from build123d import *

# Parameters (mm, degrees)
F0_R     = 3
F1_DEPTH = 10


with BuildPart() as f1:
    # F0 (on Top) → F1 (new body)
    with BuildSketch(Plane.XY):
        with BuildLine():
            ThreePointArc((4.242641, -1.5), (4.435194, -0.760959), (4.5, 0))
            ThreePointArc((4.5, 0), (4.435194, 0.760959), (4.242641, 1.5))
            ThreePointArc((4.242641, 1.5), (-4.5, 0), (4.242641, -1.5))
        make_face()
        Circle(F0_R, mode=Mode.SUBTRACT)
        with BuildLine():
            ThreePointArc((4.242641, 1.5), (4.435194, 0.760959), (4.5, 0))
            ThreePointArc((4.5, 0), (4.435194, -0.760959), (4.242641, -1.5))
            Line((4.242641, -1.5), (11.25223, -1.5))
            ThreePointArc((11.25223, -1.5), (11.161904, 0), (11.25223, 1.5))
            Line((11.25223, 1.5), (4.242641, 1.5))
        make_face()
    extrude(amount=F1_DEPTH)


solid = f1.part
Build history of the part. All positions in model axes, mm. A direction names the side the tool comes from. Give positions to 0.01 mm unless a question says otherwise; leave off trailing zeros. Write each loop counter-clockwise with the first axis right and the second up, starting at its lowest first coordinate (ties: lowest second). Pieces come first, ordered by that corner, then holes. Notation, with made-up numbers: (36.25, -2) - (60.25, -2) arc R22 cw to (60.25, 9) - close; hole circle Ø6 at (-5.5, 9). An arc over 180 degrees is marked (long way). Use one line per item in the form item = value. Start each with the question number.
1. Band-saw the part on B-B on x = 0. Write the cut outline in (y, z), plus the area to 3 significant figures.
2. Two-plate mould, pull along Y, no slides. Class faces 3 (the face through (11.16, -0.02, 4.93)), 4 (the face through (8, 1.5, 5)), 5 (the face through (3.3, 0.1, 0)): released by +Y, released by -Y, zero draft, split by the parting line, or undercut.
3. Band-saw the part on A-A on y = 0. Write the cut outline in (x, z), plus the area to 3 significant figures.
4. Band-saw the part on D-D on x = 9.25. Write the cut outline in (y, z).
5. Probe line 1 (Y direction, x = 0, z = 7.5); line 2 (X direction, y = -2.25, z = 9.75); line 3 (Y direction, x = -1, z = 6.75). List the from-to ranges inside material, lowest first. Write a range as [from, to].
6. Drop flat-ended pins along their axis: pin 1 Ø2 at (x, z) = (6, 4.5) entering from -Y; pin 2 Ø1.5 at (y, z) = (1, 1.5) entering from -X; pin 3 Ø1 at (y, z) = (-3, 4) entering from +X. Give the stop position or say it passes through.
7. 3-axis set-ups, long thin cutter, end or side, ignore diameter. For faces 1 (the face through (8, -1.5, 5)), 2 (the face through (-4.497, 0.176, 4.93)): which of +Z, -Z, +X, -X, +Y, -Y reach the whole face in a straight line?
8. Band-saw the part on C-C on z = 5.5. Write the cut outline in (x, y), plus the area to 3 significant figures.
Conclusion:
q1.outline = (-4.5, 0) - (-3, 0) - (-3, 10) - (-4.5, 10) - close; (3, 0) - (4.5, 0) - (4.5, 10) - (3, 10) - close
q1.area = 30.0 mm²
q2.face_3 = undercut
q2.face_4 = released by +Y
q2.face_5 = zero draft
q3.outline = (-4.5, 0) - (-3, 0) - (-3, 10) - (-4.5, 10) - close; (3, 0) - (11.16, 0) - (11.16, 10) - (3, 10) - close
q3.area = 96.6 mm²
q4.outline = (-1.5, 0) - (1.5, 0) - (1.5, 10) - (-1.5, 10) - close
q5.line_1 = [-4.5, -3], [3, 4.5]
q5.line_2 = [-3.9, -1.98], [1.98, 3.9]
q5.line_3 = [-4.39, -2.83], [2.83, 4.39]
q6.pin_1 = -1.5
q6.pin_2 = -4.49
q6.pin_3 = 3.74
q7.face_1 = +Z, -Z, +X, -Y
q7.face_2 = +Z, -Z
q8.outline = (4.24, -1.5) - (11.25, -1.5) arc R12.5 cw to (11.25, 1.5) - (4.24, 1.5) arc R4.5 ccw (long way) to start; hole circle Ø6 at (0, 0)
q8.area = 55.7 mm²
